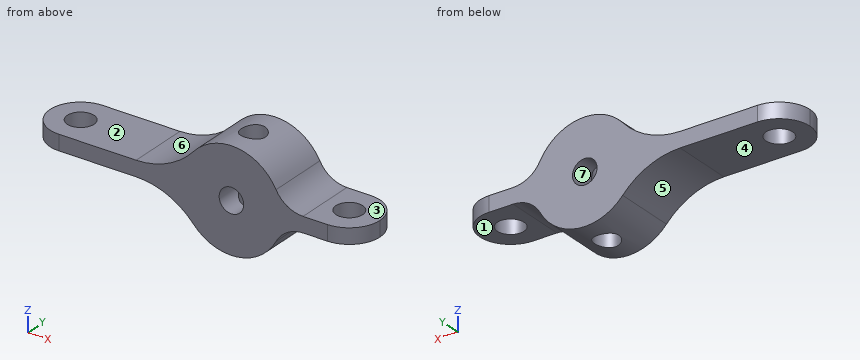
```python
from build123d import *

# Parameters (mm, degrees)
SKETCH1_R               = 1.6
BOSS_EXTRUDE1_DEPTH     = 8
CUT_EXTRUDE1_DEPTH      = 29.727549545
CUT_EXTRUDE1_DEPTH_BACK = 29.727549545
SKETCH2_R               = 1.75
SKETCH2_R_2             = 1.6
FILLET1_R               = 10
FILLET2_R               = 4
FILLET3_R               = 4


with BuildPart() as part:
    # Sketch1 → Boss-Extrude1 (new body)
    with BuildSketch(Plane(origin=(0, 0, 0), x_dir=(1, 0, 0), z_dir=(0, 1, 0))):
        with BuildLine():
            Line((-26.523802572, 1), (-6.523802572, 1))
            ThreePointArc((-6.523802572, 1), (0, 6.6), (6.523802572, 1))
            Line((6.523802572, 1), (16.523802572, 1))
            Line((16.523802572, 1), (16.523802572, -1))
            Line((16.523802572, -1), (6.523802572, -1))
            ThreePointArc((6.523802572, -1), (0, -6.6), (-6.523802572, -1))
            Line((-6.523802572, -1), (-26.523802572, -1))
            Line((-26.523802572, -1), (-26.523802572, 1))
        make_face()
        with Locations(Location((0, 0, 0), (0, 0, 270))):
            Circle(SKETCH1_R, mode=Mode.SUBTRACT)
    extrude(amount=BOSS_EXTRUDE1_DEPTH)

    # Sketch2 → Cut-Extrude1 (cut, two sides: drawn at the far end of the back side and taken through both)
    with BuildSketch(Plane.XY.offset(1).offset(-CUT_EXTRUDE1_DEPTH_BACK)):
        with BuildLine():
            ThreePointArc((-26.523802572, 4.000000071), (-25.352229672, 6.82842715), (-22.523802572, 8))
            Line((-22.523802572, 8), (-26.523802572, 8))
            Line((-26.523802572, 8), (-26.523802572, 4.000000071))
        make_face()
        with BuildLine():
            Line((-26.523802572, 0), (-22.523802572, 0))
            ThreePointArc((-22.523802572, 0), (-25.352229722, 1.171572901), (-26.523802572, 4.000000071))
            Line((-26.523802572, 4.000000071), (-26.523802572, 0))
        make_face()
        with Locations(Location((-22.523802572, 4, 0), (0, 0, 180))):
            Circle(SKETCH2_R)
        with Locations((0, 4)):
            Circle(SKETCH2_R_2)
        with Locations(Location((12.523802572, 4, 0), (0, 0, 180))):
            Circle(SKETCH2_R)
    extrude(amount=CUT_EXTRUDE1_DEPTH + CUT_EXTRUDE1_DEPTH_BACK, mode=Mode.SUBTRACT)

    # Fillet1
    fillet1_edges = [part.edges().sort_by_distance(p)[0] for p in [
        (-6.523802572, 4, 1),
        (-6.523802572, 4, -1),
    ]]
    fillet(fillet1_edges, radius=FILLET1_R)

    # Fillet2
    fillet2_edges = [part.edges().sort_by_distance(p)[0] for p in [
        (16.523802572, 0, 0),
        (16.523802572, 8, 0),
    ]]
    fillet(fillet2_edges, radius=FILLET2_R - 0.0001)  # a hair under: the kernel refuses the full size

    # Fillet3
    fillet3_edges = [part.edges().sort_by_distance(p)[0] for p in [
        (6.523802572, 4, 1),
        (6.523802572, 4, -1),
    ]]
    fillet(fillet3_edges, radius=FILLET3_R)


solid = part.part
```
Check sheet for the modelled part. Datum: model origin and axes. Units: mm. Face numbers are marked on the shaded views. A direction names the side the tool comes from. Round coordinates to 2 decimals unless told otherwise and drop trailing zeros. Write each loop counter-clockwise with the first axis right and the second up, starting at its lowest first coordinate (ties: lowest second). Pieces come first, ordered by that corner, then holes. Notation, with made-up numbers: (15.25, -25.75) -> (56.25, -25.75) arc R26 ccw to (56.25, 12.25) -> close; hole circle Ø3 at (-27.5, 3). An arc over 180 degrees is marked (long way). Put each result on its own line as item: value.
(1) Sectioned sample at A-A (y = 3). Enter the section's corners in (x, z).
Values found:
outline: (-26.4, -1) -> (-23.96, -1) -> (-23.96, 1) -> (-26.4, 1) -> close; (-21.09, -1) -> (-12.43, -1) arc R10 cw to (-4.94, -4.37) arc R6.6 ccw to (-1.25, -6.48) -> (-1.25, -1) arc R1.6 cw to (-1.25, 1) -> (-1.25, 6.48) arc R6.6 ccw to (-4.94, 4.37) arc R10 cw to (-12.43, 1) -> (-21.09, 1) -> close; (1.25, -6.48) arc R6.6 ccw to (5.82, -3.11) arc R4 cw to (9.35, -1) -> (11.09, -1) -> (11.09, 1) -> (9.35, 1) arc R4 cw to (5.82, 3.11) arc R6.6 ccw to (1.25, 6.48) -> (1.25, 1) arc R1.6 cw to (1.25, -1) -> close; (13.96, -1) -> (16.4, -1) -> (16.4, 1) -> (13.96, 1) -> close
(2) Sectioned sample at D-D (z = -3.75). Enter the section's corners in (x, y).
Values found:
outline: (-5.54, 0) -> (5.43, 0) -> (5.43, 8) -> (-5.54, 8) -> close; hole circle Ø3.2 at (0, 4)
(3) Tool access check on the marked faces 1, 2, 3 and 4. Record the directions out of +Z, -Z, +X, -X, +Y, -Y that give a thin tool (end or side, any length) a straight path to the whole face; none if there is none.
Values found:
face 1: -Z, +X, +Y, -Y
face 2: +Z, -X, +Y, -Y
face 3: +Z, +X, +Y, -Y
face 4: -Z, -X, +Y, -Y
(4) Sectioned sample at B-B (y = 0.5). Enter the section's corners in (x, z).
Values found:
outline: (-24.46, -1) -> (-12.43, -1) arc R10 cw to (-4.94, -4.37) arc R6.6 ccw to (5.82, -3.11) arc R4 cw to (9.35, -1) -> (14.46, -1) -> (14.46, 1) -> (9.35, 1) arc R4 cw to (5.82, 3.11) arc R6.6 ccw to (-4.94, 4.37) arc R10 cw to (-12.43, 1) -> (-24.46, 1) -> close; hole circle Ø3.2 at (0, 0)
(5) Sectioned sample at C-C (x = -17.5). Enter the section's corners in (y, z), plus the area to 3 significant figures.
Values found:
outline: (0, -1) -> (8, -1) -> (8, 1) -> (0, 1) -> close
area: 16.0 mm^2
(6) Mould release check, pull along Z, two halves, no side actions. Record for the marked faces 5, 6 and 7: released by +Z, released by -Z, zero draft, split by the parting line, or undercut.
Values found:
face 5: released by -Z
face 6: released by +Z
face 7: undercut
(7) Go/stop test with flat-tipped pins: pin 1 Ø2 at (x, z) = (7.5, -4.5) entering from +Y; pin 2 Ø3 at (x, y) = (6, 6) entering from -Z; pin 3 Ø1.5 at (y, z) = (4.5, -2.5) entering from -X; pin 4 Ø4.5 at (x, y) = (-22.52, 4) entering from -Z. Record where each tip stops, or that it passes through.
Values found:
pin 1: passes through
pin 2: stops at z = -4.83
pin 3: stops at x = -8.63
pin 4: stops at z = -1
(8) Material ranges on line 1 (Y direction, x = -22.5, z = 0.5); line 2 (Z direction, x = 0, y = 6.45); line 3 (Y direction, x = 0, z = 4.25), recorded low to high.
Values found:
line 1: y = 0 to 2.25, 5.75 to 8
line 2: z = -6.6 to -1.6, 1.6 to 6.6
line 3: y = 0 to 2.4, 5.6 to 8
